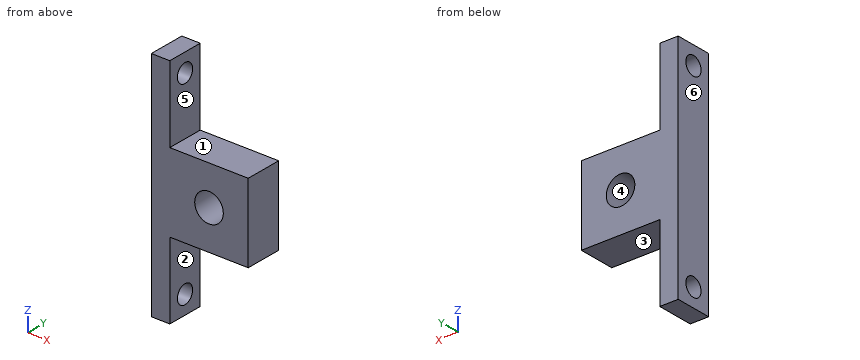
from build123d import *

# Parameters (mm, degrees)
SKETCH_1_W          = 50
SKETCH_1_H          = 8
SKETCH_1_R          = 2
EXTRUDE_1_DEPTH     = 4
SKETCH_2_W          = 17
SKETCH_2_H          = 8
EXTRUDE_2_DEPTH     = 17
SKETCH_3_R          = 3.1
CUT_EXTRUDE_1_DEPTH = 34.615472628


with BuildPart() as part:
    # 草图1 → 凸台-拉伸1 (new body)
    with BuildSketch(Plane(origin=(0, 0, 0), x_dir=(0, 0, -1), z_dir=(1, 0, 0))):
        Rectangle(SKETCH_1_W, SKETCH_1_H)
        with Locations((-21, 0)):
            Circle(SKETCH_1_R, mode=Mode.SUBTRACT)
        with Locations(Location((21, 0, 0), (0, 0, 180))):
            Circle(SKETCH_1_R, mode=Mode.SUBTRACT)
    extrude(amount=EXTRUDE_1_DEPTH)

    # 草图2 → 凸台-拉伸2 (add)
    with BuildSketch(Plane(origin=(4, 0, 0), x_dir=(0, 0, -1), z_dir=(1, 0, 0))):
        Rectangle(SKETCH_2_W, SKETCH_2_H)
    extrude(amount=EXTRUDE_2_DEPTH)

    # 草图3 → 切除-拉伸1 (cut, through all)
    with BuildSketch(Plane.XZ.offset(4)):
        with Locations(Location((12.5, 0, 0), (0, 0, 270))):
            Circle(SKETCH_3_R)
    extrude(amount=-CUT_EXTRUDE_1_DEPTH, mode=Mode.SUBTRACT)


solid = part.part
Can you work these out from the model? Positions are in its coordinate system, mm. Face numbers are marked on the shaded views. A direction names the side the tool comes from. Coordinates: 2 decimals unless noted, no trailing zeros. Write each loop counter-clockwise with the first axis right and the second up, starting at its lowest first coordinate (ties: lowest second). Pieces come first, ordered by that corner, then holes. Notation, with made-up numbers: (60.5, 83.25) -> (111.5, 83.25) arc R17 cw to (111.5, 87.25) -> close; hole circle Ø5 at (89.25, 63). An arc over 180 degrees is marked (long way). Answer as CSV lines item,"result".
1) Will these pins go through, and if not, where does the flat tip stop? P1, Ø4, axis at y = 2, z = -18, coming from the +X side; P2, Ø1.5, axis at x = 16.5, y = -3, coming from the +Z side; P3, Ø4, axis at x = 9, y = 0, coming from the -Z side.
Check result:
P1,"x = 4"
P2,"z = 8.5"
P3,"z = -8.5"
2) If we section it at C-C on y = 0.75: Please give me the cut outline in (x, z), then the cut area to 3 significant figures.
Check result:
outline,"(0, -25) -> (4, -25) -> (4, -22.85) -> (0, -22.85) -> close; (0, -19.15) -> (4, -19.15) -> (4, -8.5) -> (21, -8.5) -> (21, 8.5) -> (4, 8.5) -> (4, 19.15) -> (0, 19.15) -> close; (0, 22.85) -> (4, 22.85) -> (4, 25) -> (0, 25) -> close; hole circle Ø6.2 at (12.5, 0)"
area,"429 mm²"
3) If I drill on line 1 (X direction, y = 2.25, z = 0); line 2 (Y direction, x = 2.25, z = -21); line 3 (Z direction, x = 11.25, y = 2.75), over which ranges is the centre line in solid material (lowest first)? Write a range as from..to.
Check result:
line 1,"0..9.4, 15.6..21"
line 2,"-4..-2, 2..4"
line 3,"-8.5..-2.84, 2.84..8.5"
4) On a 3-axis mill with a long thin cutter (end or side, diameter ignored), from which of +Z, -Z, +X, -X, +Y, -Y can I reach the whole of each face in a straight line? I mean the marked faces 5 and 6. Say none if no direction works.
Check result:
face 5,"+Z, +X, +Y, -Y"
face 6,"+Z, -Z, -X, +Y, -Y"
5) If we section it at A-A on z = -21: Please give me the cut outline in (x, y), then the cut area to 3 significant figures.
Check result:
outline,"(0, -4) -> (4, -4) -> (4, -2) -> (0, -2) -> close; (0, 2) -> (4, 2) -> (4, 4) -> (0, 4) -> close"
area,"16.0 mm²"
6) If we section it at D-D on x = 18.25: Please give me the cut outline in (y, z).
Check result:
outline,"(-4, -8.5) -> (4, -8.5) -> (4, 8.5) -> (-4, 8.5) -> close"
7) If we section it at B-B on x = 12.5: Please give me the cut outline in (y, z).
Check result:
outline,"(-4, -8.5) -> (4, -8.5) -> (4, -3.1) -> (-4, -3.1) -> close; (-4, 3.1) -> (4, 3.1) -> (4, 8.5) -> (-4, 8.5) -> close"
8) If we mould it in two halves opening along Z, with no side actions, what happens to the marked faces 1, 2, 3 and 4? For each: +Z half, -Z half, draft (parallel to the pull), parting line (faces both ways), or undercut.
Check result:
face 1,"+Z half"
face 2,"draft"
face 3,"-Z half"
face 4,"undercut"
